The listing builds one solid part. Answer for the finished solid, in the listing's coordinates (mm). Give positions to 0.01 mm unless a question says otherwise; leave off trailing zeros. Write each loop counter-clockwise with the first axis right and the second up, starting at its lowest first coordinate (ties: lowest second). Pieces come first, ordered by that corner, then holes. Notation, with made-up numbers: (87, -19) -> (96, -19) arc R25 ccw to (96, -1) -> close; hole circle Ø3 at (23.25, 41.25). An arc over 180 degrees is marked (long way). One line per question, with ' | ' between items.
from build123d import *

# Parameters (mm, degrees)
SKETCH_W   = 135
SKETCH_H   = 17
SKETCH_R   = 1.65
SKETCH_R_2 = 3.4
PAD_DEPTH  = 3.125
FILLET_R   = 5


with BuildPart() as part:
    # Sketch → Pad (new body)
    with BuildSketch(Plane.XY):
        with Locations((61.5, 0)):
            Rectangle(SKETCH_W, SKETCH_H)
        Circle(SKETCH_R, mode=Mode.SUBTRACT)
        with Locations((13, 0)):
            Circle(SKETCH_R, mode=Mode.SUBTRACT)
        with Locations((26, 0)):
            Circle(SKETCH_R, mode=Mode.SUBTRACT)
        with Locations((39, 0)):
            Circle(SKETCH_R, mode=Mode.SUBTRACT)
        with Locations((52, 0)):
            Circle(SKETCH_R, mode=Mode.SUBTRACT)
        with Locations((65, 0)):
            Circle(SKETCH_R, mode=Mode.SUBTRACT)
        with Locations((91, 0)):
            Circle(SKETCH_R, mode=Mode.SUBTRACT)
        with Locations((78, 0)):
            Circle(SKETCH_R, mode=Mode.SUBTRACT)
        with Locations((117, 0)):
            Circle(SKETCH_R_2, mode=Mode.SUBTRACT)
    extrude(amount=PAD_DEPTH)

    # Fillet
    fillet_edges = [part.edges().sort_by_distance(p)[0] for p in [
        (-6, -8.5, 1.5625),
        (129, -8.5, 1.5625),
        (129, 8.5, 1.5625),
        (-6, 8.5, 1.5625),
    ]]
    fillet(fillet_edges, radius=FILLET_R)


solid = part.part
Item 1: A flat-ended cylindrical pin translates along its axis: pin 1 (2 mm diameter, centred on x = 26, y = 0, fed in from +Z). Find the tip coordinate at first contact, or state that the pin passes through.
Answers below:
pin 1: through
Item 2: Find section C-C (x = 117). Write down the section's boundary in (y, z) (3 decimals).
Answers below:
outline: (-8.5, 0) -> (-3.4, 0) -> (-3.4, 3.125) -> (-8.5, 3.125) -> close; (3.4, 0) -> (8.5, 0) -> (8.5, 3.125) -> (3.4, 3.125) -> close
Item 3: Find section B-B (z = 2.35). Count the separate pieces of the cut face and the enclosed holes in it, then the cut area to 3 significant figures.
Answers below:
separate pieces: 1 | enclosed holes: 9 | area: 2,170 mm²
Item 4: Determine the mould class of faces 1 (the face through (76.35, 0.07, 1.54)), 2 (the face through (-1.216, 1.115, 1.541)), 3 (the face through (-4.57, -7, 1.58)), 4 (the face through (-6, 0, 2)) for opening direction Y: pulls with the +Y half, pulls with the -Y half, needs draft (parallel to the pull), parting line crosses it, or undercut.
Answers below:
face 1: undercut | face 2: undercut | face 3: pulls with the -Y half | face 4: needs draft
Item 5: Find section A-A (x = 78). Write down the section's boundary in (y, z) (3 decimals).
Answers below:
outline: (-8.5, 0) -> (-1.65, 0) -> (-1.65, 3.125) -> (-8.5, 3.125) -> close; (1.65, 0) -> (8.5, 0) -> (8.5, 3.125) -> (1.65, 3.125) -> close
Item 6: Consider line 1 (Y direction, x = 26, z = 1.7); line 2 (Y direction, x = 1.5, z = 0.8); line 3 (X direction, y = 2.25, z = 2.6). Determine where each line is inside the solid, lowest interval first. Write a range as [from, to].
Answers below:
line 1: [-8.5, -1.65], [1.65, 8.5] | line 2: [-8.5, -0.69], [0.69, 8.5] | line 3: [-6, 114.45], [119.55, 129]
